from build123d import *

# Parameters (mm, degrees)
CUT_EXTRUDE1_DEPTH        = 12
M3X0_5_TAPPED_HOLE1_D     = 2.5
M3X0_5_TAPPED_HOLE1_DEPTH = 8.5
M3X0_5_TAPPED_HOLE1_TIP   = 0.751075774
CUT_EXTRUDE2_DEPTH        = 2


with BuildPart() as part:
    # Sketch1 → MainBody (revolve)
    with BuildSketch(Plane.XY):
        Polygon((0, 0), (0, 8.625), (-4, 8.625), (-4, 5), (-12, 5), (-12, 17.25), (-14, 17.25), (-14, 5), (-15, 5), (-15, 17.25), (-45.8, 17.25), (-45.8, 18.5), (-67.7, 18.5), (-67.7, 0), align=None)
    revolve(axis=Axis((-80.111398028, 0, 0), (1, 0, 0)))

    # Sketch3 → SmallBoss (revolve)
    with BuildSketch(Plane.XY):
        Polygon((-67.7, 7), (-67.7, 13), (-73.5, 13), (-73.5, 10), (-88.7, 10), (-88.7, 7), align=None)
    revolve(axis=Axis((0, 7, 0), (-1, 0, 0)))

    # Sketch4 → Cut-Extrude1 (cut)
    with BuildSketch(Plane.ZY.offset(88.7)):
        with BuildLine():
            Line((-2.75, 5.801042119), (-2.75, 8.198957881))
            ThreePointArc((-2.75, 8.198957881), (-3, 7), (-2.75, 5.801042119))
        make_face()
        with BuildLine():
            ThreePointArc((3, 7), (2.936835031, 7.612372436), (2.75, 8.198957881))
            Line((2.75, 8.198957881), (2.75, 5.801042119))
            ThreePointArc((2.75, 5.801042119), (2.936835031, 6.387627564), (3, 7))
        make_face()
    extrude(amount=-CUT_EXTRUDE1_DEPTH, mode=Mode.SUBTRACT)

    # M3x0.5 Tapped Hole1
    with Locations(Plane.ZY.offset(67.7)):
        with Locations((7.75, 13.423393759), (15.5, 0), (7.75, -13.423393759), (-7.75, -13.423393759), (-15.5, 0), (-7.75, 13.423393759)):
            Hole(M3X0_5_TAPPED_HOLE1_D / 2, depth=M3X0_5_TAPPED_HOLE1_DEPTH)
            with Locations((0, 0, -(M3X0_5_TAPPED_HOLE1_DEPTH + M3X0_5_TAPPED_HOLE1_TIP / 2))):  # 118° drill point
                Cone(0, M3X0_5_TAPPED_HOLE1_D / 2, M3X0_5_TAPPED_HOLE1_TIP, mode=Mode.SUBTRACT)

    # Sketch9 → Cut-Extrude2 (cut)
    with BuildSketch(Plane.ZY.offset(67.7)):
        with BuildLine():
            ThreePointArc((-9.324839925, 6.385470704), (-3.342227597, -10.796128493), (11.301631552, 0))
            ThreePointArc((11.301631552, 0), (10.796128493, 3.342227597), (9.324839925, 6.385470704))
            ThreePointArc((9.324839925, 6.385470704), (0, -2.345067463), (-9.324839925, 6.385470704))
        make_face()
    extrude(amount=-CUT_EXTRUDE2_DEPTH, mode=Mode.SUBTRACT)


solid = part.part
Source: CAD feature listing. Evaluate the final solid. Frame: model axes, mm. A direction names the side the tool comes from. Round coordinates to 2 decimals unless told otherwise and drop trailing zeros. Order: outer loops, then holes, each group sorted by start corner. A loop starts at its lowest first (then second) coordinate and runs counter-clockwise, first axis right, second up. Notation, with made-up numbers: (58.25, 2) - (90.25, 2) arc R20 cw to (90.25, 30) - close; hole circle Ø5 at (-5, 6). An arc over 180 degrees is marked (long way). Use a Markdown table: item, result. Add a question column.
1. Section query A-A (x = -35.5). Return the cut outline in (y, z).
2. Mould query, pull axis Z, two halves, no side actions, for faces 1 (the conical face through (-58.58, -13.28, -7.91)), 2 (the conical face through (-58.58, -13.28, 7.59)), 3 (the flat face through (-45.8, -5, 17)), 4 (the cylindrical face through (-56.9, -4.01, -18.06)). Classes: +Z half, -Z half, draft (parallel to the pull), parting line (faces both ways), or undercut.
3. Section query C-C (x = -79). Return the cut outline in (y, z).
4. Line query: probe 1 along Z at (x, y) = (-65.5, 0); probe 2 along X at (y, z) = (0, 6); probe 3 along X at (y, z) = (-7, 7). Output: solid intervals per line, ascending.
5. Set-up query: faces 5 (the flat face through (-12, -4, -4)), 6 (the flat face through (-83, 7, -2.75)), 7 (the flat face through (-83, 7, 2.75)), 8 (the cylindrical face through (-63.39, -12.58, 8.67)). Return all of +Z, -Z, +X, -X, +Y, -Y with unobstructed straight access to the full face (end or side cutting, diameter ignored); none if empty.
6. First-contact query: pin 1 (4 mm diameter, centred on y = 13.42, z = -7.75, fed in from +X); pin 2 (1 mm diameter, centred on x = -12.5, z = 8.5, fed in from -Y); pin 3 (12 mm diameter, centred on x = -35, y = -7, fed in from +Z). Flat tips, straight axial feed; report the tip coordinate or a pass-through.
7. Section query D-D (x = -5.5). Return the cut outline in (y, z).
Derived:
| question | item | result |
|---|---|---|
| 1 | outline | circle Ø34.5 at (0, 0) |
| 2 | face 1 | undercut |
| 2 | face 2 | undercut |
| 2 | face 3 | draft |
| 2 | face 4 | parting line |
| 3 | outline | (5.8, -2.75) - (8.2, -2.75) arc R3 ccw to (8.2, 2.75) - (5.8, 2.75) arc R3 ccw to start |
| 4 | probe 1 | -18.5 to -16.75, -14.25 to 14.25, 16.75 to 18.5 |
| 4 | probe 2 | -67.7 to -15, -14 to -12, -4 to 0 |
| 4 | probe 3 | -65.7 to -15, -14 to -12 |
| 5 | face 5 | none |
| 5 | face 6 | -Z, -X, +Y, -Y |
| 5 | face 7 | +Z, -X, +Y, -Y |
| 5 | face 8 | -X |
| 6 | pin 1 | x = -12 |
| 6 | pin 2 | y = -15.28 |
| 6 | pin 3 | z = 17.22 |
| 7 | outline | circle Ø10 at (0, 0) |
